Input: part model. Units: mm. Frame: model coordinates. Face numbers are marked on the shaded views. A direction names the side the tool comes from. Round coordinates to 2 decimals unless told otherwise and drop trailing zeros. Loops run counter-clockwise (first coordinate to the right, second up) from the corner with the lowest first, then second, coordinate; pieces in that order, holes last.
1) Section D-D, the plane z = 39.5. Return loops of the section in (x, y) (3 decimals), and give its area (3 significant figures).
2) First-contact query: pin 1 (8 mm diameter, centred on y = 13.5, z = 35, fed in from -X) (3 decimals); pin 2 (17.5 mm diameter, centred on x = -16, z = 8, fed in from -Y); pin 3 (13 mm diameter, centred on x = -39, y = 34.5, fed in from +Z); pin 4 (2 mm diameter, centred on x = -24, z = 22, fed in from -Y). Flat tips, straight axial feed; report the tip coordinate or a pass-through.
3) Section C-C, the plane y = 10.5. Return loops of the section in (x, z) (3 decimals).
4) Section A-A, the plane x = -42. Return loops of the section in (y, z) (3 decimals).
5) Access query for the marked faces 1, 2 and 3. Directions: +Z, -Z, +X, -X, +Y, -Y. A direction counts if a zero-diameter tool reaches every point of the face in a straight line with its end or side. Return the directions, or none.
6) Ray query, line 1 along Y through (x, z) = (-27.5, 26) (3 decimals); line 2 along X through (y, z) = (33, 7); line 3 along Z through (x, y) = (-30, 34). Return the intervals inside material, ascending.
7) Section B-B, the plane z = 13. Return loops of the section in (x, y).
8) Draft query along Z for the marked faces 4, 5 and 6. Return one class per face: pulls with the +Z half, pulls with the -Z half, needs draft (parallel to the pull), parting line crosses it, or undercut.
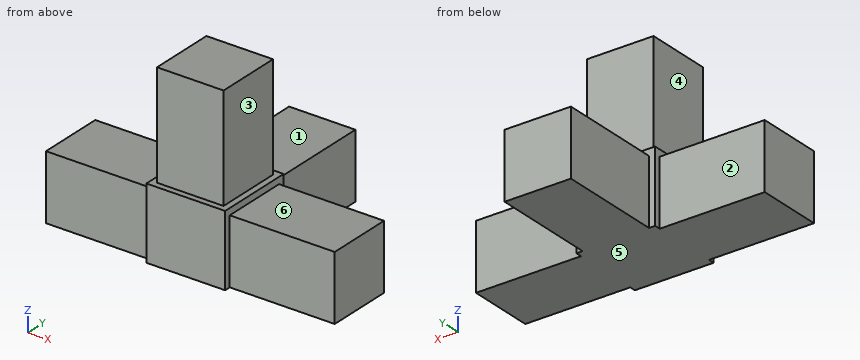
from build123d import *

# Parameters (mm, degrees)
F1_DEPTH = 15.85
F3_DEPTH = 1.6
F4_W     = 16.1
F4_H     = 16.1
F5_DEPTH = 25.4


with BuildPart() as f1:
    # F0 (on Top) → F1 (new body)
    with BuildSketch(Plane.XY):
        Polygon((-25.4, 1.5), (0, 1.5), (0, 17.55), (-25.4, 17.55), (-25.4, 19.05), (-26.9, 19.05), (-26.9, 44.45), (-42.95, 44.45), (-42.95, 19.05), (-44.45, 19.05), (-44.45, 17.55), (-69.85, 17.55), (-69.85, 1.5), (-44.45, 1.5), (-44.45, 0), (-25.4, 0), align=None)
    extrude(amount=F1_DEPTH)

    # F2 (on face) → F3 (join)
    with BuildSketch(Plane.XY.offset(15.85)):
        Polygon((-42.95, 19.05), (-44.45, 19.05), (-44.45, 17.55), (-44.45, 1.5), (-44.45, 0), (-25.4, 0), (-25.4, 1.5), (-25.4, 17.55), (-25.4, 19.05), (-26.9, 19.05), align=None)
    extrude(amount=F3_DEPTH)

    # F4 (on face) → F5 (join)
    with BuildSketch(Plane.XY.offset(17.45)):
        with Locations((-34.925, 9.525)):
            Rectangle(F4_W, F4_H)
    extrude(amount=F5_DEPTH)


solid = f1.part
Final values:
1. outline: (-42.975, 1.475) - (-26.875, 1.475) - (-26.875, 17.575) - (-42.975, 17.575) - close
1. area: 259 mm2
2. pin 1: stops at x = -42.975
2. pin 2: stops at y = 1.5
2. pin 3: stops at z = 15.85
2. pin 4: passes through
3. outline: (-69.85, 0) - (0, 0) - (0, 15.85) - (-25.4, 15.85) - (-25.4, 17.45) - (-26.875, 17.45) - (-26.875, 42.85) - (-42.975, 42.85) - (-42.975, 17.45) - (-44.45, 17.45) - (-44.45, 15.85) - (-69.85, 15.85) - close
4. outline: (0, 0) - (44.45, 0) - (44.45, 15.85) - (19.05, 15.85) - (19.05, 17.45) - (17.575, 17.45) - (17.575, 42.85) - (1.475, 42.85) - (1.475, 17.45) - (0, 17.45) - close
5. face 1: +Z, +X, -X, +Y
5. face 2: +Z, -Z, -X, +Y
5. face 3: +Z, +X, +Y, -Y
6. line 1: y = 1.475 to 17.575
6. line 2: x = -42.95 to -26.9
6. line 3: z = 0 to 15.85
7. outline: (-69.85, 1.5) - (-44.45, 1.5) - (-44.45, 0) - (-25.4, 0) - (-25.4, 1.5) - (0, 1.5) - (0, 17.55) - (-25.4, 17.55) - (-25.4, 19.05) - (-26.9, 19.05) - (-26.9, 44.45) - (-42.95, 44.45) - (-42.95, 19.05) - (-44.45, 19.05) - (-44.45, 17.55) - (-69.85, 17.55) - close
8. face 4: needs draft
8. face 5: pulls with the -Z half
8. face 6: pulls with the +Z half
